Design review of the part shown in the three views and the two pictorial views. Dimensions are in mm from the part's minimum x, y and z. Coordinates: 2 decimals unless noted, no trailing zeros. Write each loop counter-clockwise with the first axis right and the second up, starting at its lowest first coordinate (ties: lowest second). Pieces come first, ordered by that corner, then holes. Notation, with made-up numbers: (-32, 71) -> (12, 71) arc R21 cw to (12, 81) -> close; hole circle Ø1 at (67.5, 81.25). An arc over 180 degrees is marked (long way). Write item = value, one per line. Start each with the question number.
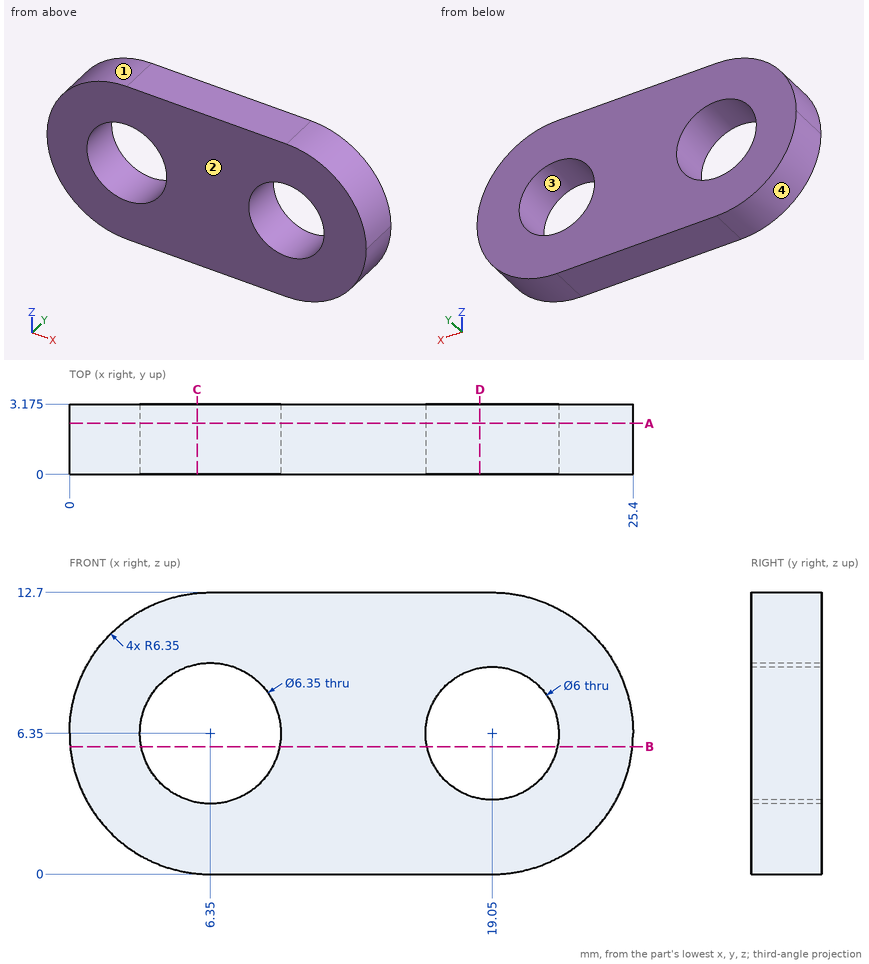
(1) Mouldability with a two-part tool opening along Z and no side actions: class the marked faces 1, 2, 3 and 4 as pulls with the +Z half, pulls with the -Z half, needs draft (parallel to the pull), parting line crosses it, or undercut.
(2) Take a section at B-B, the plane z = 5.75. State the section outline as (x, y) points (1 decimal), then the cut area to 3 significant figures.
(3) Take a section at D-D, the plane x = 18.5. State the section outline as (y, z) points (3 decimals).
(4) For pin 1 Ø5.5 at (x, z) = (19.05, 6.35) entering from +Y, flat-tipped, find the tip position at first contact; note if it passes through.
(5) Take a section at A-A, the plane y = 2.3. Count the separate pieces of the cut face and the enclosed holes in it, then the cut area to 3 significant figures.
(6) Take a section at C-C, the plane x = 5.75. State the section outline as (y, z) points (1 decimal), then the cut area to 3 significant figures.
(7) For line 1 (X direction, y = 0.8, z = 6.35) (3 decimals); line 2 (X direction, y = 2.6, z = 4.25); line 3 (Z direction, x = 18.5, y = 2.65), list the stretches that pass through material, from the lowest coordinate up.
Report:
q1.face_1 = pulls with the +Z half
q1.face_2 = needs draft
q1.face_3 = undercut
q1.face_4 = pulls with the -Z half
q2.outline = (0, 0) -> (3.2, 0) -> (3.2, 3.2) -> (0, 3.2) -> close; (9.5, 0) -> (16.1, 0) -> (16.1, 3.2) -> (9.5, 3.2) -> close; (22, 0) -> (25.4, 0) -> (25.4, 3.2) -> (22, 3.2) -> close
q2.area = 42.0 mm2
q3.outline = (0, 0) -> (3.175, 0) -> (3.175, 3.401) -> (0, 3.401) -> close; (0, 9.299) -> (3.175, 9.299) -> (3.175, 12.7) -> (0, 12.7) -> close
q4.pin_1 = through
q5.separate_pieces = 1
q5.enclosed_holes = 2
q5.area = 228 mm2
q6.outline = (0, 0) -> (3.2, 0) -> (3.2, 3.2) -> (0, 3.2) -> close; (0, 9.5) -> (3.2, 9.5) -> (3.2, 12.7) -> (0, 12.7) -> close
q6.area = 20.3 mm2
q7.line_1 = 0 to 3.175, 9.525 to 16.05, 22.05 to 25.4
q7.line_2 = 0.36 to 3.97, 8.73 to 16.91, 21.19 to 25.04
q7.line_3 = 0 to 3.4, 9.3 to 12.7
